Autodesk Inventor part; units mm, degrees
ref_plane "YZ Plane" through (0, 0, 0) normal (1, 0, 0) x (0, 1, 0)
ref_plane "XZ Plane" through (0, 0, 0) normal (0, 1, 0) x (-1, 0, 0)
ref_plane "XY Plane" through (0, 0, 0) normal (0, 0, 1) x (1, 0, 0)
sketch "Sketch1" plane through (0, 0, 0) normal (0, 0, 1) x (1, 0, 0)
  line L0 (0, 0) -> (6.35, 0)
  line L1 (6.35, 0) -> (6.35, 5)
  line L2 (0, 5) -> (0, 0)
  line L3 (12.7, 0) -> (19.05, 0)
  line L4 (19.05, 0) -> (19.05, 5)
  line L5 (12.7, 5) -> (12.7, 0)
  line L6 (25.4, 0) -> (31.75, 0)
  line L7 (31.75, 0) -> (31.75, 5)
  line L8 (25.4, 5) -> (25.4, 0)
  line L9 (38.1, 0) -> (44.45, 0)
  line L10 (44.45, 0) -> (44.45, 5)
  line L11 (38.1, 5) -> (38.1, 0)
  line L12 (50.8, 0) -> (57.15, 0)
  line L13 (57.15, 0) -> (57.15, 5)
  line L14 (50.8, 5) -> (50.8, 0)
  line L15 (63.5, 0) -> (69.85, 0)
  line L16 (69.85, 0) -> (69.85, 5)
  line L17 (63.5, 5) -> (63.5, 0)
  line L18 (76.2, 5) -> (76.2, 30.4)
  line L19 (76.2, 30.4) -> (0, 30.4)
  line L20 (0, 30.4) -> (0, 5)
  line L21 (6.35, 5) -> (12.7, 5)
  line L22 (19.05, 5) -> (25.4, 5)
  line L23 (31.75, 5) -> (38.1, 5)
  line L24 (44.45, 5) -> (50.8, 5)
  line L25 (57.15, 5) -> (63.5, 5)
  line L26 (69.85, 5) -> (76.2, 5)
  dimension "d3" = 6.35
  dimension "d4" = 5
  dimension "d7" = 12.7
  dimension "d12" = 76.2
  dimension "d13" = 25.4
extrude "Extrusion1" add sketch "Sketch1" along normal blind 5
sketch "Sketch2" plane through (0, 0, 5) normal (0, 0, 1) x (1, 0, 0)
  line L0 (71.12, 27.5) -> (58.12, 27.5)
  line L1 (58.12, 27.5) -> (58.12, 7.9)
  line L2 (58.12, 7.9) -> (71.12, 7.9)
  line L3 (71.12, 7.9) -> (71.12, 27.5)
  line L4 (76.2, 17.7) -> (0.6797, 17.7)
  line L5 (76.2, 5) -> (76.2, 30.4)
  point P0 (0, 0)
  point P1 (71.12, 17.7)
  dimension "d16" = 13
  dimension "d17" = 19.6
  dimension "d20" = 5.08
extrude "Switch" cut sketch "Sketch2" against normal blind 5
sketch "Sketch3" plane through (0, 0, 5) normal (0, 0, 1) x (1, 0, 0)
  circle A0 centre (46.69, 17.7) radius 2.5
  line L0 (76.2, 5) -> (76.2, 30.4) construction
  line L1 (58.12, 7.9) -> (58.12, 27.5) construction
  line L2 (76.2, 17.7) -> (0, 17.7) construction
  line L3 (0, 30.4) -> (0, 0) construction
  dimension "d23" = 5
  dimension "d24" = 11.43
extrude "LED" cut sketch "Sketch3" against normal blind 5
sketch "Sketch4" plane through (0, 0, 5) normal (0, 0, 1) x (1, 0, 0)
  circle A0 centre (33.02, 17.7) radius 3.6
  line L0 (76.2, 5) -> (76.2, 30.4) construction
  line L1 (76.2, 17.7) -> (0, 17.7) construction
  circle A1 centre (20.32, 17.7) radius 3.6
  circle A2 centre (7.62, 17.7) radius 3.6
  line L2 (0, 30.4) -> (0, 0)
  dimension "d27" = 7.2
  dimension "d28" = 7.2
  dimension "d29" = 7.2
  dimension "d30" = 12.7
  dimension "d31" = 12.7
  dimension "d33" = 7.62
extrude "Buttons" cut sketch "Sketch4" against normal blind 5
equation "\"d4\" = hardboard_thickness"
equation "\"d14\" = hardboard_thickness"
equation "\"d21\" = hardboard_thickness"
equation "\"d25\" = hardboard_thickness"
equation "\"d34\" = hardboard_thickness"
equation "\"m3_heat_set_insert\" = 4"
equation "\"m3_clearance\" = 3.4"
equation "\"m3_heat_set_depth\" = 7"
equation "\"robot_diameter\" = 354"
equation "\"hardboard_thickness\" = 5"
properties part number "control_panel"
Source: CAD feature listing. Evaluate the final solid. Frame: model axes, mm. A direction names the side the tool comes from. Give positions to 0.01 mm unless a question says otherwise; leave off trailing zeros. Loops run counter-clockwise (first coordinate to the right, second up) from the corner with the lowest first, then second, coordinate; pieces in that order, holes last. Notation, with made-up numbers: (-32.75, 42) - (-25.75, 42) arc R36 ccw to (-25.75, 79) - close; hole circle Ø9 at (55.25, 11). An arc over 180 degrees is marked (long way). Use CSV: the item, a comma, the result in double quotes. Start each with the question number.
1. Pin query (flat end, axial travel): pin 1 (1.5 mm diameter, centred on y = 3, z = 3.5, fed in from +X); pin 2 (1.5 mm diameter, centred on x = 47, z = 3.5, fed in from -Y). Return the tip coordinate at first contact, or that it passes through.
2. Draft query along X for faces 1 (the flat face through (0, 15, 2)), 2 (the cylindrical face through (21.981, 14.506, 2.535)), 3 (the flat face through (38, 15, 5)). Return one class per face: +X half, -X half, draft (parallel to the pull), parting line (faces both ways), or undercut.
3. Reachability of faces 4 (the flat face through (69.85, 2, 2)), 5 (the flat face through (6.35, 2, 2)), 6 (the flat face through (16, 0, 2)) from +Z, -Z, +X, -X, +Y, -Y: full face, straight path, thin tool, end or side. Return the list, or none.
4. Ray query, L1, parallel to Y at x = 7.62, z = 2.1; L2, parallel to X at y = 22, z = 3.4; L3, parallel to Y at x = 46.69, z = 1.6. Return the intervals inside material, ascending.
5. Section C-C (y = 9). Output: boundary loops of the cut face in (x, z).
6. Section B-B (y = 17.7). Output: boundary loops of the cut face in (x, z), then the cut area to 3 significant figures.
7. Section D-D (z = 1.7). Count the separate pieces of the cut face and the enclosed holes in it, then the cut area to 3 significant figures.
8. Section A-A (x = 7.62). Output: boundary loops of the cut face in (y, z).
Response:
1,pin 1,"x = 69.85"
1,pin 2,"y = 5"
2,face 1,"-X half"
2,face 2,"undercut"
2,face 3,"draft"
3,face 4,"+Z, -Z, +X, -Y"
3,face 5,"+Z, -Z, -Y"
3,face 6,"+Z, -Z, +X, -X, -Y"
4,L1,"5 to 14.1, 21.3 to 30.4"
4,L2,"0 to 58.12, 71.12 to 76.2"
4,L3,"5 to 15.2, 20.2 to 30.4"
5,outline,"(0, 0) - (58.12, 0) - (58.12, 5) - (0, 5) - close; (71.12, 0) - (76.2, 0) - (76.2, 5) - (71.12, 5) - close"
6,outline,"(0, 0) - (4.02, 0) - (4.02, 5) - (0, 5) - close; (11.22, 0) - (16.72, 0) - (16.72, 5) - (11.22, 5) - close; (23.92, 0) - (29.42, 0) - (29.42, 5) - (23.92, 5) - close; (36.62, 0) - (44.19, 0) - (44.19, 5) - (36.62, 5) - close; (49.19, 0) - (58.12, 0) - (58.12, 5) - (49.19, 5) - close; (71.12, 0) - (76.2, 0) - (76.2, 5) - (71.12, 5) - close"
6,area,"183 mm²"
7,separate pieces,"1"
7,enclosed holes,"5"
7,area,"1,730 mm²"
8,outline,"(5, 0) - (14.1, 0) - (14.1, 5) - (5, 5) - close; (21.3, 0) - (30.4, 0) - (30.4, 5) - (21.3, 5) - close"
